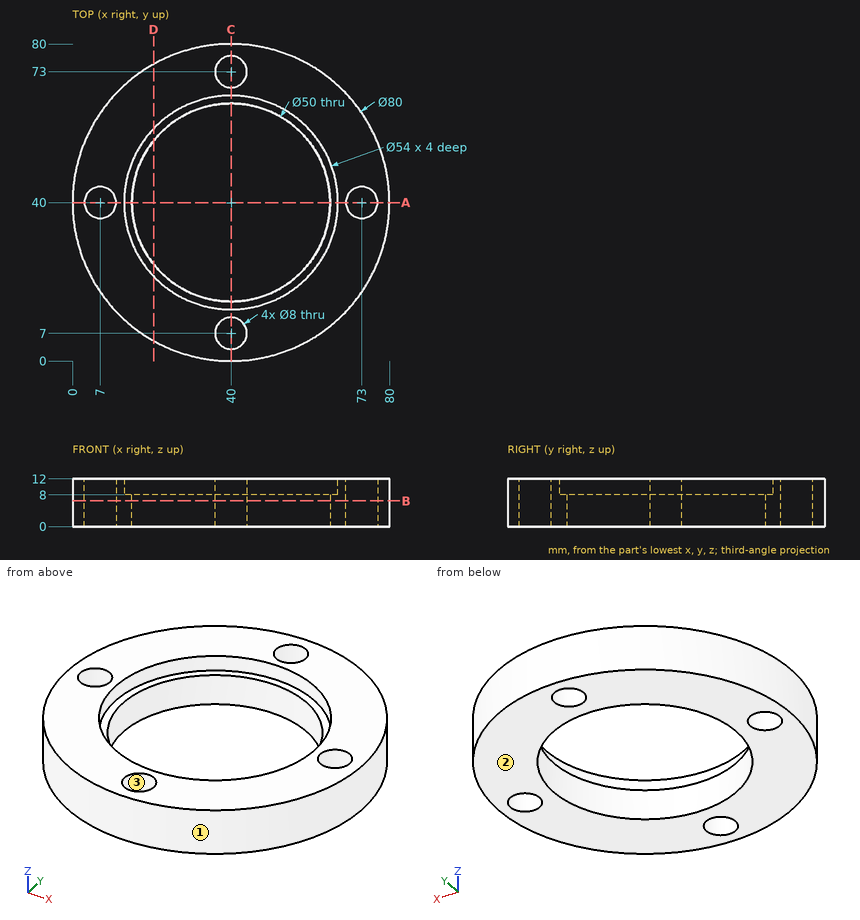
Could you check a few things on this drawing? It's one solid part, dimensions in mm from its lowest x, y, z. Coordinates: 2 decimals unless noted, no trailing zeros. Loops run counter-clockwise (first coordinate to the right, second up) from the corner with the lowest first, then second, coordinate; pieces in that order, holes last. Notation, with made-up numbers: (4, -28) - (23, -28) arc R34 cw to (23, 3) - close; hole circle Ø3 at (-15.75, 68). An arc over 180 degrees is marked (long way). Answer as a JSON object with one key per item and string values. Group by question number.
Item 1: If we section it at A-A (y = 40): List the corners of the cut face in (x, z) for me, plus the area to 3 significant figures.
Item 2: If we section it at B-B (z = 6.5): List the corners of the cut face in (x, y) for me.
Item 3: If we section it at D-D (x = 20.5): List the corners of the cut face in (y, z) for me, plus the area to 3 significant figures.
Item 4: If I drill on L1, parallel to Y at x = 40, z = 3.75; L2, parallel to Y at x = 40, z = 11.15; L3, parallel to X at y = 39, z = 11.75, over which ranges is the centre line in solid material (lowest first)? Write a range as from..to.
Item 5: If we mould it in two halves opening along Y, with no side actions, what happens to the marked faces 1, 2 and 3? For each: released by +Y, released by -Y, zero draft, split by the parting line, or undercut.
Item 6: For pin 1 (6 mm diameter, centred on x = 43, z = 9, fed in from +Y); pin 2 (1.5 mm diameter, centred on y = 47.5, z = 4, fed in from -X); pin 3 (5 mm diameter, centred on x = 51, z = 9.5, fed in from +Y); pin 4 (10.5 mm diameter, centred on x = 73, y = 40, fed in from -Z), each with a flat end and sliding along its axis, tell me the tip position at first contact or that it passes through.
Returned:
{
 "1": {"outline": "(0, 0) - (3, 0) - (3, 12) - (0, 12) - close; (11, 0) - (15, 0) - (15, 8) - (13, 8) - (13, 12) - (11, 12) - close; (65, 0) - (69, 0) - (69, 12) - (67, 12) - (67, 8) - (65, 8) - close; (77, 0) - (80, 0) - (80, 12) - (77, 12) - close", "area": "152 mm²"},
 "2": {"outline": "circle Ø80 at (40, 40); hole circle Ø8 at (7, 40); hole circle Ø50 at (40, 40); hole circle Ø8 at (40, 7); hole circle Ø8 at (40, 73); hole circle Ø8 at (73, 40)"},
 "3": {"outline": "(5.08, 0) - (24.36, 0) - (24.36, 8) - (21.33, 8) - (21.33, 12) - (5.08, 12) - close; (55.64, 0) - (74.92, 0) - (74.92, 12) - (58.67, 12) - (58.67, 8) - (55.64, 8) - close", "area": "438 mm²"},
 "4": {"L1": "y = 0..3, 11..15, 65..69, 77..80", "L2": "y = 0..3, 11..13, 67..69, 77..80", "L3": "x = 0.01..3.13, 10.87..13.02, 66.98..69.13, 76.87..79.99"},
 "5": {"face 1": "split by the parting line", "face 2": "zero draft", "face 3": "undercut"},
 "6": {"pin 1": "stops at y = 80", "pin 2": "stops at x = 0.57", "pin 3": "stops at y = 79.09", "pin 4": "stops at z = 0"}
}
